```python
from build123d import *

# Parameters (mm, degrees)
F0_W     = 25.4
F0_H     = 6.35
F1_DEPTH = 76.2
F2_W     = 25.4
F2_H     = 3.175
F3_DEPTH = 6.35
F4_W     = 19.05
F4_H     = 3.175
F5_DEPTH = 6.35


with BuildPart() as f1:
    # F0 (on Right) → F1 (new body)
    with BuildSketch(Plane.YZ):
        Rectangle(F0_W, F0_H)
    extrude(amount=F1_DEPTH)

    # F2 (on face) → F3 (join)
    with BuildSketch(Plane.XZ.offset(12.7)):
        with Locations((38.1, 1.5875)):
            Rectangle(F2_W, F2_H)
    extrude(amount=F3_DEPTH)

    # F4 (on face) → F5 (join)
    with BuildSketch(Plane(origin=(0, 12.7, 0), x_dir=(-1, 0, 0), z_dir=(0, 1, 0))):
        with Locations((-60.325, 1.5875)):
            Rectangle(F4_W, F4_H)
        with Locations((-15.875, 1.5875)):
            Rectangle(F4_W, F4_H)
    extrude(amount=F5_DEPTH)


solid = f1.part
```
Here's how the part is built. I have some questions about the finished solid (model axes, mm). A direction names the side the tool comes from. Give positions to 0.01 mm unless a question says otherwise; leave off trailing zeros. Loops run counter-clockwise (first coordinate to the right, second up) from the corner with the lowest first, then second, coordinate; pieces in that order, holes last. Notation, with made-up numbers: M 64,10 L 99,10 A13 ccw 99,35 Z; hole C -16.5,45.25 d8. An arc over 180 degrees is marked long. Return JSON: item names as keys, results as strings.
Item 1: I'm going to push flat-ended pins straight in: pin 1 Ø2.5 at (y, z) = (15, 2) entering from -X; pin 2 Ø1.9 at (x, z) = (22, 0.5) entering from -Y; pin 3 Ø3.5 at (y, z) = (-14.5, 1.5) entering from +X. Where does each tip first touch, or does it pass through?
A:
{"pin 1": "stops at x = 6.35", "pin 2": "stops at y = -12.7", "pin 3": "stops at x = 50.8"}
Item 2: Imagine slicing it at D-D on y = -16. List the corners of the cut face in (x, z) for me (3 decimals).
A:
{"outline": "M 25.4,0 L 50.8,0 L 50.8,3.175 L 25.4,3.175 Z"}
Item 3: On a 3-axis mill with a long thin cutter (end or side, diameter ignored), from which of +Z, -Z, +X, -X, +Y, -Y can I reach the whole of each face in a straight line? I mean faces 1 (the flat face through (50.8, -16, 2)), 2 (the flat face through (38, -16, 0)), 3 (the flat face through (69.85, 16, 2)), 4 (the flat face through (25.4, 16, 2)), 5 (the flat face through (60, 16, 0)). Say none if no direction works.
A:
{"face 1": "+Z, -Z, +X, -Y", "face 2": "-Z, +X, -X, -Y", "face 3": "+Z, -Z, +X, +Y", "face 4": "+Z, -Z, +Y", "face 5": "-Z, +X, -X, +Y"}
Item 4: Imagine slicing it at A-A on y = 14. List the corners of the cut face in (x, z) for me (3 decimals).
A:
{"outline": "M 6.35,0 L 25.4,0 L 25.4,3.175 L 6.35,3.175 Z; M 50.8,0 L 69.85,0 L 69.85,3.175 L 50.8,3.175 Z"}
Item 5: Thinking about a two-plate mould opening in X: for faces 6 (the flat face through (38, -12.7, -1)), 7 (the flat face through (38, 12.7, -1)), 8 (the flat face through (25.4, -16, 2)), which applies, released by +X, released by -X, zero draft, split by the parting line, or undercut?
A:
{"face 6": "zero draft", "face 7": "undercut", "face 8": "released by -X"}
Item 6: Imagine slicing it at B-B on z = 0.75. List the corners of the cut face in (x, y) for me, then the cut area to 3 significant figures.
A:
{"outline": "M 0,-12.7 L 25.4,-12.7 L 25.4,-19.05 L 50.8,-19.05 L 50.8,-12.7 L 76.2,-12.7 L 76.2,12.7 L 69.85,12.7 L 69.85,19.05 L 50.8,19.05 L 50.8,12.7 L 25.4,12.7 L 25.4,19.05 L 6.35,19.05 L 6.35,12.7 L 0,12.7 Z", "area": "2,340 mm^2"}
Item 7: Please list where these lines run through material, in increasing order: line 1 (Y direction, x = 23.5, z = -0.75); line 2 (Y direction, x = 54.5, z = 2); line 3 (Z direction, x = 57, y = 13.5) (3 decimals).
A:
{"line 1": "y = -12.7 to 12.7", "line 2": "y = -12.7 to 19.05", "line 3": "z = 0 to 3.175"}
Item 8: Imagine slicing it at C-C on x = 29.5. List the corners of the cut face in (y, z) for me (3 decimals).
A:
{"outline": "M -19.05,0 L -12.7,0 L -12.7,-3.175 L 12.7,-3.175 L 12.7,3.175 L -19.05,3.175 Z"}
